Could you check a few things on this model? Use its own coordinates, in mm. A direction names the side the tool comes from. Coordinates: 2 decimals unless noted, no trailing zeros. Write each loop counter-clockwise with the first axis right and the second up, starting at its lowest first coordinate (ties: lowest second). Pieces come first, ordered by that corner, then holes.
```python
from build123d import *

# Parameters (mm, degrees)
CUT_EXTRUDE1_DEPTH = 2.794
CIRPATTERN1_COUNT  = 10
SKETCH3_R          = 4
CUT_EXTRUDE2_DEPTH = 13.7
SKETCH4_R          = 2.25
CUT_EXTRUDE3_DEPTH = 10
SKETCH5_R          = 2.25
CUT_EXTRUDE4_DEPTH = 10


with BuildPart() as part:
    # Sketch1 → Revolve2 (revolve)
    with BuildSketch(Plane.XY):
        Polygon((0, 0), (10.274515829, 0), (11.676645231, -0.247233244), (11.676645231, -2.546766756), (10.274515829, -2.794), (6.35, -2.794), (6.35, -12.2), (5.85, -12.7), (0, -12.7), align=None)
    revolve(axis=Axis((0, 0, 0), (0, -1, 0)))

    # Sketch2 → Cut-Extrude1 (cut)
    with BuildSketch(Plane(origin=(0, 0, 0), x_dir=(1, 0, 0), z_dir=(0, 1, 0))):
        with BuildLine():
            Line((1.428941916, 9.449515829), (2.551819083, 11.394396132))
            ThreePointArc((2.551819083, 11.394396132), (0, 11.676645231), (-2.551819083, 11.394396132))
            Line((-2.551819083, 11.394396132), (-1.428941916, 9.449515829))
            ThreePointArc((-1.428941916, 9.449515829), (0, 8.624515829), (1.428941916, 9.449515829))
        make_face()
    cut_extrude1 = extrude(amount=-CUT_EXTRUDE1_DEPTH, mode=Mode.SUBTRACT)

    # CirPattern1: Cut-Extrude1 ×10 about axis
    cirpattern1_axis = Axis((0, 0, 0), (0, 1, 0))
    for i in range(1, CIRPATTERN1_COUNT):
        add(cut_extrude1.rotate(cirpattern1_axis, i * 360 / CIRPATTERN1_COUNT), mode=Mode.SUBTRACT)

    # Sketch3 → Cut-Extrude2 (cut, through all)
    with BuildSketch(Plane.XZ.offset(12.7)):
        Circle(SKETCH3_R)
    extrude(amount=-CUT_EXTRUDE2_DEPTH, mode=Mode.SUBTRACT)

    # Sketch4 → Cut-Extrude3 (cut)
    with BuildSketch(Plane(origin=(0, 0, 0), x_dir=(0, 0, -1), z_dir=(1, 0, 0))):
        with Locations((0, -7.747)):
            Circle(SKETCH4_R)
    extrude(amount=-CUT_EXTRUDE3_DEPTH, mode=Mode.SUBTRACT)

    # Sketch5 → Cut-Extrude4 (cut)
    with BuildSketch(Plane.XY):
        with Locations((0, -7.497)):
            Circle(SKETCH5_R)
    extrude(amount=-CUT_EXTRUDE4_DEPTH, mode=Mode.SUBTRACT)


solid = part.part
```
1. If we mould it in two halves opening along X, with no side actions, what happens to faces 1 (the face through (5.05, -1.38, -6.99)), 2 (the face through (8.9, -0.125, 6.44)), 3 (the face through (2.15, -6.439, 3.373)), 4 (the face through (-5, -2.794, 5))? For each: pulls with the +X half, pulls with the -X half, needs draft (parallel to the pull), parting line crosses it, or undercut.
Verdict:
face 1: undercut
face 2: pulls with the +X half
face 3: undercut
face 4: needs draft
2. I want a section at A-A on x = 0. Please give me the cut outline in (y, z), plus the area to 3 significant figures.
Verdict:
outline: (-12.7, -5.85) - (-12.2, -6.35) - (-9.75, -6.35) - (-9.75, -4) - (-12.7, -4) - close; (-12.7, 4) - (0, 4) - (0, 8.62) - (-2.79, 8.62) - (-2.79, 6.35) - (-12.2, 6.35) - (-12.7, 5.85) - close; (-5.25, -6.35) - (-2.79, -6.35) - (-2.79, -8.62) - (0, -8.62) - (0, -4) - (-5.25, -4) - close
area: 61.6 mm2
3. For pin 1 (5 mm diameter, centred on x = -7.5, y = -10, fed in from +Z); pin 2 (3.5 mm diameter, centred on y = -7.747, z = 0, fed in from -X); pin 3 (1.5 mm diameter, centred on y = -1.5, z = -8.5, fed in from -X), each with a flat end and sliding along its axis, tell me the tip position at first contact or that it passes through.
Verdict:
pin 1: stops at z = 3.91
pin 2: stops at x = 3.6
pin 3: stops at x = -4.49
4. I want a section at C-C on y = -7. Please give me the cut outline in (x, z).
Verdict:
outline: (-5.98, -2.12) arc R6.35 ccw to (-2.19, -5.96) - (-2.19, -3.34) arc R4 cw to (-3.39, -2.12) - close; (-5.98, 2.12) - (-3.39, 2.12) arc R4 cw (long way) to (2.19, -3.34) - (2.19, -5.96) arc R6.35 ccw (long way) to start
5. On a 3-axis mill with a long thin cutter (end or side, diameter ignored), from which of +Z, -Z, +X, -X, +Y, -Y can I reach the whole of each face in a straight line? I mean faces 5 (the face through (7.75, -1.377, 7.268)), 6 (the face through (6.057, -7.563, 1.907)), 7 (the face through (-8.875, -0.125, 6.474)), 8 (the face through (-5.089, -1.377, -6.963)), 9 (the face through (-9.286, -1.377, -5.102)). Say none if no direction works.
Verdict:
face 5: +Z, +Y, -Y
face 6: -Y
face 7: +Z, -X, +Y
face 8: +Y, -Y
face 9: -X, +Y, -Y
6. I want a section at B-B on z = 0. Please give me the cut outline in (x, y), plus the area to 3 significant figures.
Verdict:
outline: (-11.68, -2.55) - (-10.27, -2.79) - (-6.35, -2.79) - (-6.35, -5.5) - (-4, -5.5) - (-4, 0) - (-10.27, 0) - (-11.68, -0.25) - close; (-6.35, -12.2) - (-5.85, -12.7) - (-4, -12.7) - (-4, -10) - (-6.35, -10) - close; (4, -12.7) - (5.85, -12.7) - (6.35, -12.2) - (6.35, -2.79) - (10.27, -2.79) - (11.68, -2.55) - (11.68, -0.25) - (10.27, 0) - (4, 0) - close
area: 77.9 mm2
7. Please list where these lines run through material, in increasing order: line 1 along X through (y, z) = (-1.25, 7.5); line 2 along X through (y, z) = (-2.5, 10); line 3 along Y through (x, z) = (-5.75, -1.5).
Verdict:
line 1: x = -8.95 to -8.27, -4.6 to 4.6, 8.27 to 8.95
line 2: x = -4.56 to -1.75, 1.75 to 4.56
line 3: y = -12.61 to -9.42, -6.07 to 0
